The listing builds one solid part. Answer for the finished solid, in the listing's coordinates (mm). A direction names the side the tool comes from. Round coordinates to 2 decimals unless told otherwise and drop trailing zeros. Loops run counter-clockwise (first coordinate to the right, second up) from the corner with the lowest first, then second, coordinate; pieces in that order, holes last. Notation, with made-up numbers: (79, 50) - (94, 50) arc R27 ccw to (94, 79) - close; hole circle Ø7 at (61, 30.5). An arc over 180 degrees is marked (long way). One line per item, written item: value.
```python
from build123d import *

# Parameters (mm, degrees)
F0_W      = 2
F0_H      = 10.5
F0_H_2    = 2
F0_W_2    = 5
F1_DEPTH  = 16.1
F0_H_3    = 21
F0_W_3    = 30.5
F2_DEPTH  = 5.6
F3_DEPTH  = 5.6
F4_R      = 2
F22_DEPTH = 1
F23_DEPTH = 25
F24_DEPTH = 1
F25_DEPTH = 25
F26_R     = 0.99999
F27_W     = 10
F27_H     = 2.5
F28_DEPTH = 15


# Not quite as in the source:
# - a fillet or chamfer is up to 0.001 mm smaller than in the source, because OpenCascade refuses the exact size


with BuildPart() as f1:
    # F0 (on Top) → F1 (new body)
    with BuildSketch(Plane.XY):
        with Locations((53.5, 28.25)):
            Rectangle(F0_W, F0_H)
        with Locations((53.5, 34.5)):
            Rectangle(F0_W, F0_H_2)
        Polygon((52.5, 23), (49.5, 23), (49.5, 21), (54.5, 21), (54.5, 23), align=None)
        Polygon((47.5, 23), (47.5, 2), (49.5, 2), (49.5, 21), (49.5, 23), align=None)
        with Locations((48.5, 1)):
            Rectangle(F0_W, F0_H_2)
        with Locations((45, 1)):
            Rectangle(F0_W_2, F0_H_2)
        with Locations((50, 34.5)):
            Rectangle(F0_W_2, F0_H_2)
    extrude(amount=F1_DEPTH)



with BuildPart() as f1b:
    # F0 (on Top) → F1, piece 2 (new body)
    with BuildSketch(Plane.XY):
        with Locations((6, 34.5)):
            Rectangle(F0_W, F0_H_2)
        Polygon((5, 25), (5, 23), (7, 23), (7, 33.5), (5, 33.5), align=None)
        Polygon((0, 25), (0, 23), (2, 23), (5, 23), (5, 25), align=None)
        with Locations((1, 12.5)):
            Rectangle(F0_W, F0_H_3)
        with Locations((1, 1)):
            Rectangle(F0_W, F0_H_2)
        with Locations((4.5, 1)):
            Rectangle(F0_W_2, F0_H_2)
        with Locations((9.5, 34.5)):
            Rectangle(F0_W_2, F0_H_2)
    extrude(amount=F1_DEPTH)


with BuildPart() as f1_1:
    add(f1.part)

    add(f1b.part)  # F2 merges F1b
    # F0 (on Top) → F2 (join)
    with BuildSketch(Plane.XY):
        with Locations((27.25, 34.5)):
            Rectangle(F0_W_3, F0_H_2)
        with Locations((45, 34.5)):
            Rectangle(F0_W_2, F0_H_2)
        with Locations((9.5, 1)):
            Rectangle(F0_W_2, F0_H_2)
        Polygon((2, 23), (2, 2), (7, 2), (7, 23), (5, 23), align=None)
        Polygon((7, 23), (7, 2), (12, 2), (12, 5), (12, 7), (12, 23), align=None)
        with Locations((9.5, 28.25)):
            Rectangle(F0_W_2, F0_H)
        Polygon((42.5, 33.5), (42.5, 23), (47.5, 23), (49.5, 23), (52.5, 23), (52.5, 33.5), (47.5, 33.5), align=None)
        Polygon((42.5, 5), (42.5, 2), (47.5, 2), (47.5, 23), (42.5, 23), (42.5, 7), align=None)
    extrude(amount=F2_DEPTH)

    # F0 (on Top) → F3 (join)
    with BuildSketch(Plane.XY):
        with Locations((27.25, 6)):
            Rectangle(F0_W_3, F0_H_2)
    extrude(amount=F3_DEPTH)

    # F4
    f4_edges = [f1_1.edges().sort_by_distance(p)[0] for p in [
        (0, 0, 8.05),
        (0, 25, 8.05),
        (5, 35.5, 8.05),
        (54.5, 35.5, 8.05),
        (54.5, 21, 8.05),
        (49.5, 0, 8.05),
    ]]
    fillet(f4_edges, radius=F4_R)

    # F18 (on 3pt) + F19 (on 3pt) → F22 (join)
    with BuildSketch(Plane.YZ.offset(2)):
        Polygon((4.75, 11.85), (4.75, 9.85), (7.25, 9.85), (9.75, 9.85), (9.75, 11.85), (7.25, 11.85), align=None)
        Polygon((15.25, 11.85), (15.25, 9.85), (17.75, 9.85), (20.25, 9.85), (20.25, 11.85), (17.75, 11.85), align=None)
    with BuildSketch(Plane.YZ.offset(7)):
        Polygon((26.25, 11.85), (26.25, 9.85), (28.75, 9.85), (31.25, 9.85), (31.25, 11.85), (28.75, 11.85), align=None)
    extrude(amount=F22_DEPTH)

    # F18 (on 3pt) + F19 (on 3pt) → F23 (cut)
    with BuildSketch(Plane.YZ.offset(2)):
        with BuildLine():
            ThreePointArc((18.25, 12.35), (17.3964466094, 12.7035533906), (17.75, 11.85))
            ThreePointArc((17.75, 11.85), (18.1035533906, 11.9964466094), (18.25, 12.35))
        make_face()
        with BuildLine():
            ThreePointArc((18.25, 9.35), (18.1035533906, 9.7035533906), (17.75, 9.85))
            ThreePointArc((17.75, 9.85), (17.3964466094, 8.9964466094), (18.25, 9.35))
        make_face()
        with BuildLine():
            ThreePointArc((7.75, 9.35), (7.6035533906, 9.7035533906), (7.25, 9.85))
            ThreePointArc((7.25, 9.85), (6.8964466094, 8.9964466094), (7.75, 9.35))
        make_face()
        with BuildLine():
            ThreePointArc((7.75, 12.35), (6.8964466094, 12.7035533906), (7.25, 11.85))
            ThreePointArc((7.25, 11.85), (7.6035533906, 11.9964466094), (7.75, 12.35))
        make_face()
    with BuildSketch(Plane.YZ.offset(7)):
        with BuildLine():
            ThreePointArc((29.25, 12.35), (28.3964466094, 12.7035533906), (28.75, 11.85))
            ThreePointArc((28.75, 11.85), (29.1035533906, 11.9964466094), (29.25, 12.35))
        make_face()
        with BuildLine():
            ThreePointArc((29.25, 9.35), (29.1035533906, 9.7035533906), (28.75, 9.85))
            ThreePointArc((28.75, 9.85), (28.3964466094, 8.9964466094), (29.25, 9.35))
        make_face()
    extrude(amount=-F23_DEPTH, mode=Mode.SUBTRACT)

    # F20 (on 3pt) + F21 (on 3pt) → F24 (join)
    with BuildSketch(Plane(origin=(47.5, 0, 0), x_dir=(0, -1, 0), z_dir=(-1, 0, 0))):
        Polygon((-20.5, 11.85), (-20.5, 9.85), (-18, 9.85), (-15.5, 9.85), (-15.5, 11.85), (-18, 11.85), align=None)
        Polygon((-9.75, 11.85), (-9.75, 9.85), (-7.25, 9.85), (-4.75, 9.85), (-4.75, 11.85), (-7.25, 11.85), align=None)
    with BuildSketch(Plane.YZ.offset(52.5)):
        Polygon((26.25, 11.85), (26.25, 9.85), (28.75, 9.85), (31.25, 9.85), (31.25, 11.85), (28.75, 11.85), align=None)
    extrude(amount=F24_DEPTH, dir=(-1, 0, 0))

    # F21 (on 3pt) + F20 (on 3pt) → F25 (cut)
    with BuildSketch(Plane.YZ.offset(52.5)):
        with BuildLine():
            ThreePointArc((29.25, 12.35), (28.3964466094, 12.7035533906), (28.75, 11.85))
            ThreePointArc((28.75, 11.85), (29.1035533906, 11.9964466094), (29.25, 12.35))
        make_face()
        with BuildLine():
            ThreePointArc((29.25, 9.35), (29.1035533906, 9.7035533906), (28.75, 9.85))
            ThreePointArc((28.75, 9.85), (28.3964466094, 8.9964466094), (29.25, 9.35))
        make_face()
    with BuildSketch(Plane(origin=(47.5, 0, 0), x_dir=(0, -1, 0), z_dir=(-1, 0, 0))):
        with BuildLine():
            ThreePointArc((-17.5, 12.35), (-18.3535533906, 12.7035533906), (-18, 11.85))
            ThreePointArc((-18, 11.85), (-17.6464466094, 11.9964466094), (-17.5, 12.35))
        make_face()
        with BuildLine():
            ThreePointArc((-17.5, 9.35), (-17.6464466094, 9.7035533906), (-18, 9.85))
            ThreePointArc((-18, 9.85), (-18.3535533906, 8.9964466094), (-17.5, 9.35))
        make_face()
        with BuildLine():
            ThreePointArc((-6.75, 12.35), (-7.6035533906, 12.7035533906), (-7.25, 11.85))
            ThreePointArc((-7.25, 11.85), (-6.8964466094, 11.9964466094), (-6.75, 12.35))
        make_face()
        with BuildLine():
            ThreePointArc((-6.75, 9.35), (-6.8964466094, 9.7035533906), (-7.25, 9.85))
            ThreePointArc((-7.25, 9.85), (-7.6035533906, 8.9964466094), (-6.75, 9.35))
        make_face()
    extrude(amount=F25_DEPTH, dir=(1, 0, 0), mode=Mode.SUBTRACT)

    # F26 (radius 1 in the source; OpenCascade refuses exactly that, so slightly less here)
    f26_edges = [f1_1.edges().sort_by_distance(p)[0] for p in [
        (3, 7.25, 11.85),
        (3, 7.25, 9.85),
        (3, 17.75, 11.85),
        (3, 17.75, 9.85),
        (8, 28.75, 11.85),
        (8, 28.75, 9.85),
        (46.5, 18, 9.85),
        (46.5, 7.25, 9.85),
        (46.5, 7.25, 11.85),
        (46.5, 18, 11.85),
        (51.5, 28.75, 11.85),
        (51.5, 28.75, 9.85),
    ]]
    fillet(f26_edges, radius=F26_R)

    # F27 (on face) → F28 (cut)
    with BuildSketch(Plane.XZ.offset(-5)):
        with Locations((32.5, 1.25)):
            Rectangle(F27_W, F27_H)
    extrude(amount=-F28_DEPTH, mode=Mode.SUBTRACT)


solid = f1_1.part
```
1) Each of these flat-tipped pins is pushed along its axis until it touches: pin 1 Ø0.9 at (y, z) = (7.25, 9.35) entering from -X; pin 2 Ø4 at (y, z) = (1.5, 4) entering from +X; pin 3 Ø2.5 at (x, z) = (45, 12) entering from +Y. Where does it stop, or does it pass through?
Final values:
pin 1: through
pin 2: x = 49.5
pin 3: y = 2
2) A cutting plane is placed at A-A on x = 40.5. Give the vertices of the cut face in (y, z).
Final values:
outline: (5, 0) - (7, 0) - (7, 5.6) - (5, 5.6) - close; (33.5, 0) - (35.5, 0) - (35.5, 5.6) - (33.5, 5.6) - close
3) A cutting plane is placed at D-D on y = 22. Give the vertices of the cut face in (x, z), and give its area (3 significant figures).
Final values:
outline: (0, 0) - (12, 0) - (12, 5.6) - (2, 5.6) - (2, 16.1) - (0, 16.1) - close; (42.5, 0) - (54.23, 0) - (54.23, 16.1) - (47.5, 16.1) - (47.5, 5.6) - (42.5, 5.6) - close
area: 225 mm2
4) For faces 5 (the flat face through (42.5, 1, 6)), 6 (the flat face through (27.5, 6, 1)), 7 (the flat face through (12, 34, 11)), 8 (the flat face through (4, 23, 11)), 9 (the flat face through (49.5, 11, 8)), determine the directions among +Z, -Z, +X, -X, +Y, -Y from which every point of the face is accessible in a straight line to the end or side of a thin tool.
Final values:
face 5: +Z, -Z, -Y
face 6: -Z, -Y
face 7: +Z, +Y, -Y
face 8: +Z
face 9: +Z, -Z, +X, -Y
5) For a pull along Y with two mould halves and no side action, classify faces 1 (the cylindrical face through (53.9, 21.57, 8.16)), 2 (the flat face through (27, 7, 3)), 3 (the flat face through (1.5, 20.5, 16.1)), 4 (the flat face through (50, 23, 11)) as released by +Y, released by -Y, zero draft, split by the parting line, or undercut.
Final values:
face 1: released by -Y
face 2: undercut
face 3: zero draft
face 4: undercut
6) Consider L1, parallel to Z at x = 5.95, y = 28.75; L2, parallel to Y at x = 3.5, z = 12; L3, parallel to Y at x = 48.35, z = 12.35. Determine where each line is inside the solid, lowest interval first.
Final values:
L1: 0 to 8.85, 9.85 to 11.85, 12.85 to 16.1
L2: 0 to 2, 23 to 25
L3: 0.19 to 6.75, 7.75 to 17.5, 18.5 to 23, 33.5 to 35.5
